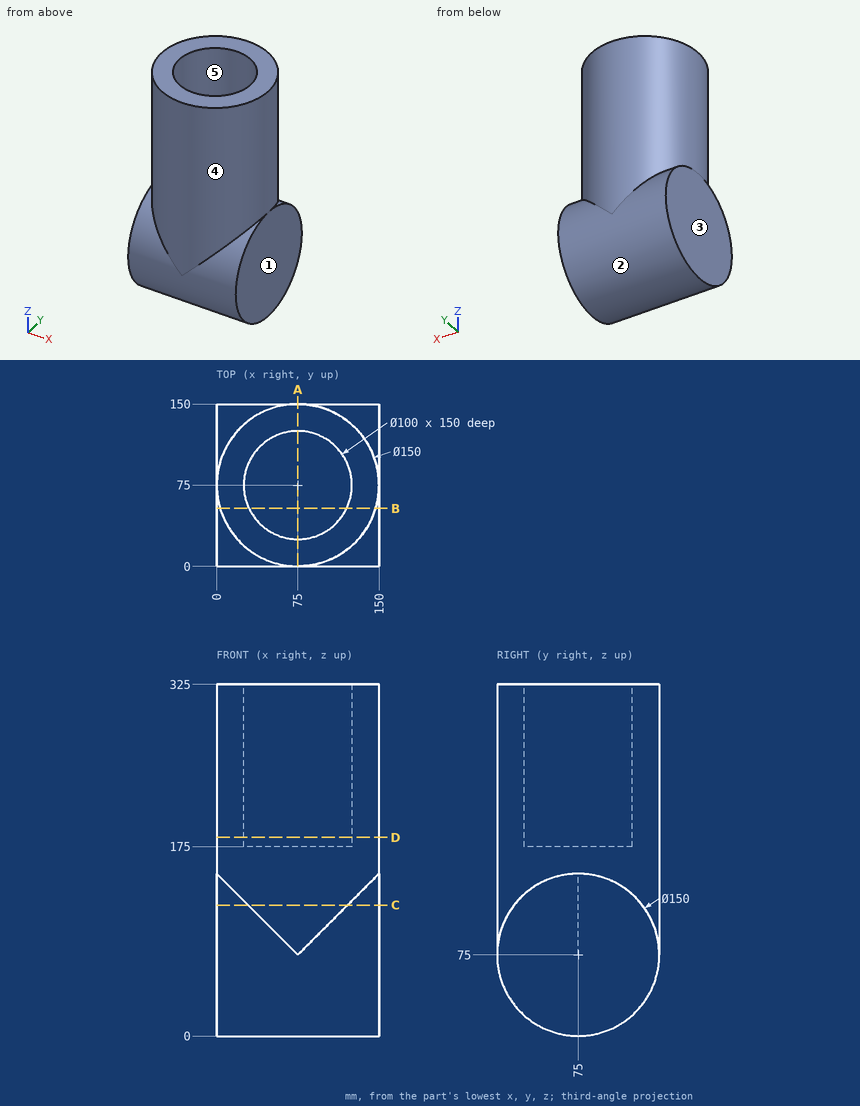
Geometry check sheet. Reference: drawing and pictorial views, mm from the part's lowest x, y, z. A direction names the side the tool comes from. Give positions to 0.01 mm unless a question says otherwise; leave off trailing zeros. Order: outer loops, then holes, each group sorted by start corner. A loop starts at its lowest first (then second) coordinate and runs counter-clockwise, first axis right, second up. Notation, with made-up numbers: (80.25, -39.75) - (93.25, -39.75) arc R23 ccw to (93.25, -17.75) - close; hole circle Ø6 at (71.5, 65). An arc over 180 degrees is marked (long way). Use one line per item in the form item = value.
1) Draft check along Y on the marked faces 3, 4 and 5. Enter one of: released by +Y, released by -Y, zero draft, split by the parting line, or undercut.
Working result:
face_3 = zero draft
face_4 = split by the parting line
face_5 = undercut
2) Sectioned sample at A-A (x = 75). Record the boundary of the cut face in (y, z), and give its area (3 significant figures).
Working result:
outline = (0, 75) arc R75 ccw to (150, 75) - (150, 325) - (125, 325) - (125, 175) - (25, 175) - (25, 325) - (0, 325) - close
area = 31,300 mm^2
3) Access from +Z, -Z, +X, -X, +Y, -Y to the whole of each face (thin tool, end or side, straight path). Record for the marked faces 1 and 2.
Working result:
face_1 = +Z, -Z, +X, +Y, -Y
face_2 = none
4) Sectioned sample at B-B (y = 53.5). Record the boundary of the cut face in (x, z), and give its area (3 significant figures).
Working result:
outline = (0, 3.15) - (150, 3.15) - (150, 146.85) - (146.85, 146.85) - (146.85, 325) - (120.14, 325) - (120.14, 175) - (29.86, 175) - (29.86, 325) - (3.15, 325) - (3.15, 146.85) - (0, 146.85) - close
area = 33,600 mm^2
5) Sectioned sample at C-C (z = 121). Record the boundary of the cut face in (x, y).
Working result:
outline = (0, 15.76) - (29, 15.76) arc R75 ccw to (121, 15.76) - (150, 15.76) - (150, 134.24) - (121, 134.24) arc R75 ccw to (29, 134.24) - (0, 134.24) - close
6) Material ranges on probe 1 along Y at (x, z) = (75, 233); probe 2 along Y at (x, z) = (93, 311.5); probe 3 along X at (y, z) = (45.5, 268), recorded low to high. Write a range as from..to.
Working result:
probe_1 = 0..25, 125..150
probe_2 = 2.19..28.35, 121.65..147.81
probe_3 = 6.05..34.63, 115.37..143.95
7) Sectioned sample at D-D (z = 183.5). Record the boundary of the cut face in (x, y), and give its area (3 significant figures).
Working result:
outline = circle Ø150 at (75, 75); hole circle Ø100 at (75, 75)
area = 9,820 mm^2
8) Depth check by flat-ended pin: pin 1 Ø3 at (x, z) = (50, 70.5) entering from -Y; pin 2 Ø3 at (x, z) = (119, 152) entering from -Y; pin 3 Ø6 at (x, y) = (73.5, 24) entering from -Z. Enter the tip coordinate at first touch or a pass-through.
Working result:
pin_1 = 0.06
pin_2 = 13.2
pin_3 = 17.37
